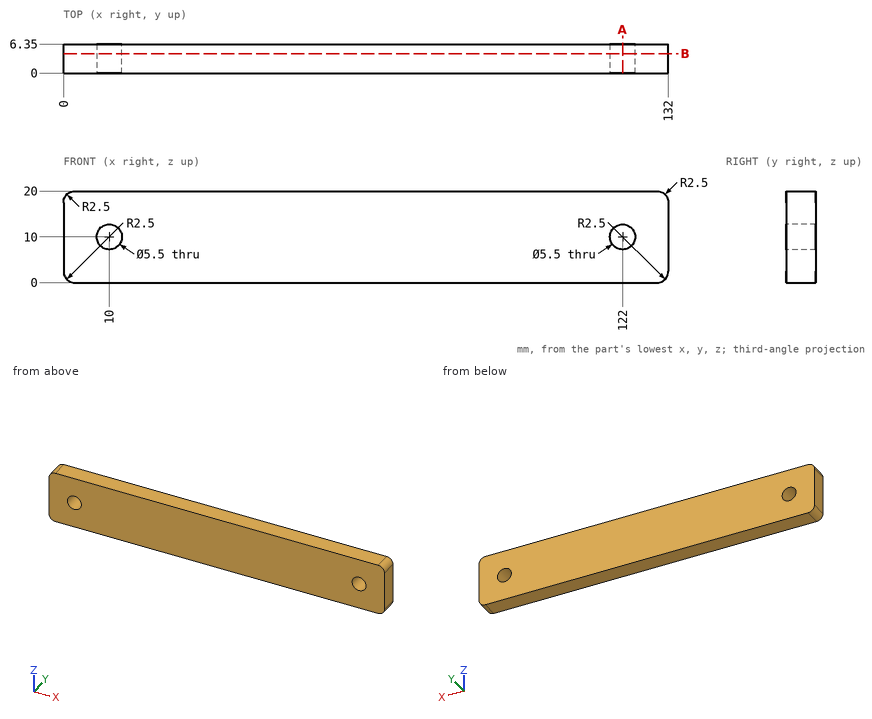
For this review, use the dimensioned drawing (mm, ordinates from the lowest corner) and the shaded views. Coordinates: 2 decimals unless noted, no trailing zeros. Order: outer loops, then holes, each group sorted by start corner. A loop starts at its lowest first (then second) coordinate and runs counter-clockwise, first axis right, second up. Notation, with made-up numbers: (29.25, -13.75) - (61.25, -13.75) arc R22 cw to (61.25, -2.75) - close; hole circle Ø9 at (14, -34). An arc over 180 degrees is marked (long way). Answer in a Markdown table with one row per item.
(1) Consider section B-B on y = 4.25. State the section outline as (x, z) points.
Checked values:
| item | result |
|---|---|
| outline | (0, 2.5) arc R2.5 ccw to (2.5, 0) - (129.5, 0) arc R2.5 ccw to (132, 2.5) - (132, 17.5) arc R2.5 ccw to (129.5, 20) - (2.5, 20) arc R2.5 ccw to (0, 17.5) - close; hole circle Ø5.5 at (10, 10); hole circle Ø5.5 at (122, 10) |
(2) Clearance check with flat-ended pins moving along their axes: pin 1 (3.5 mm diameter, centred on x = 10, z = 10, fed in from +Y); pin 2 (8 mm diameter, centred on x = 96.5, z = 13.5, fed in from -Y). State where each tip first meets the part, or that it passes through.
Checked values:
| item | result |
|---|---|
| pin 1 | through |
| pin 2 | y = 0 |
(3) Wall thickness on line 1 along X through (y, z) = (4.5, 10); line 2 along Z through (x, y) = (10, 4.75); line 3 along X through (y, z) = (6, 9): over which ranges is each line inside the solid? List them lowest first. Write a range as from..to.
Checked values:
| item | result |
|---|---|
| line 1 | 0..7.25, 12.75..119.25, 124.75..132 |
| line 2 | 0..7.25, 12.75..20 |
| line 3 | 0..7.44, 12.56..119.44, 124.56..132 |
(4) Consider section A-A on x = 122. State the section outline as (y, z) points.
Checked values:
| item | result |
|---|---|
| outline | (0, 0) - (6.35, 0) - (6.35, 7.25) - (0, 7.25) - close; (0, 12.75) - (6.35, 12.75) - (6.35, 20) - (0, 20) - close |
